from build123d import *

# Parameters (mm, degrees)
F0_W        = 304.8
F0_H        = 304.8
F0_R        = 139.7
F1_DEPTH    = 63.5
F3_D        = 6.35
F2_W        = 38.1
F2_H        = 38.1
F2_R        = 1.5875
F4_DEPTH    = 25.4
F5_T1_DEPTH = 825.5


# Not quite as in the source:
# - a fillet or chamfer that OpenCascade refuses, or shapes differently, is made with other operations: its cross-section is extruded or revolved along the edge and cut away or added


with BuildPart() as f1:
    # F0 (on Top) → F1 (new body)
    with BuildSketch(Plane.XY):
        Rectangle(F0_W, F0_H)
        Circle(F0_R, mode=Mode.SUBTRACT)
    extrude(amount=F1_DEPTH)

    # F3 (through all)
    with Locations(Plane(origin=(0, 152.4, 0), x_dir=(-1, 0, 0), z_dir=(0, 1, 0))):
        with Locations((0, 31.75)):
            Hole(F3_D / 2)

    # F2 (on face) → F4 (cut)
    with BuildSketch(Plane(origin=(0, 152.4, 0), x_dir=(-1, 0, 0), z_dir=(0, 1, 0))):
        with Locations((0, 31.75)):
            Rectangle(F2_W, F2_H)
        with Locations((0, 31.75)):
            Circle(F2_R, mode=Mode.SUBTRACT)
    extrude(amount=-F4_DEPTH, mode=Mode.SUBTRACT)

    # F5: fillet of radius 152.4 on 4 edges, made by hand

    # F5_s2 → F5_t1 (cut)
    with BuildSketch(Plane.XY.offset(-381)):
        with BuildLine():
            ThreePointArc((0, 152.4), (-107.7630734528, 107.7630734528), (-152.4, 0))
            Line((-152.4, 0), (-152.4, 152.4))
            Line((-152.4, 152.4), (0, 152.4))
        make_face()
        with BuildLine():
            ThreePointArc((152.4, 0), (107.7630734528, 107.7630734528), (0, 152.4))
            Line((0, 152.4), (152.4, 152.4))
            Line((152.4, 152.4), (152.4, 0))
        make_face()
        with BuildLine():
            ThreePointArc((152.4, 0), (107.7630734528, -107.7630734528), (0, -152.4))
            Line((0, -152.4), (152.4, -152.4))
            Line((152.4, -152.4), (152.4, 0))
        make_face()
        with BuildLine():
            ThreePointArc((0, -152.4), (-107.7630734528, -107.7630734528), (-152.4, 0))
            Line((-152.4, 0), (-152.4, -152.4))
            Line((-152.4, -152.4), (0, -152.4))
        make_face()
    extrude(amount=F5_T1_DEPTH, mode=Mode.SUBTRACT)


solid = f1.part
Read the model definition and answer for the solid it produces. Units are mm, in the model's axes. A direction names the side the tool comes from. Round coordinates to 2 decimals unless told otherwise and drop trailing zeros. Order: outer loops, then holes, each group sorted by start corner. A loop starts at its lowest first (then second) coordinate and runs counter-clockwise, first axis right, second up. Notation, with made-up numbers: (2.5, -12.5) - (24.5, -12.5) arc R19 cw to (24.5, -7.5) - close; hole circle Ø7 at (65, 38.5). An arc over 180 degrees is marked (long way). Use one line per item in the form item = value. Start each with the question number.
(1) For faces 1 (the face through (67, -123, 0)), 2 (the face through (0, 145, 50.8)), determine the directions among +Z, -Z, +X, -X, +Y, -Y from which every point of the face is accessible in a straight line to the end or side of a thin tool.
(2) Find the intervals of material crossed by line 1 along Z through (x, y) = (0, -145) (3 decimals); line 2 along X through (y, z) = (3, 20); line 3 along X through (y, z) = (-86, 54), in increasing order. Write a range as from..to.
(3) The part is cut by section C-C (z = 58.5). Give the vertices of the cut face in (x, y), then the cut area to 3 significant figures.
(4) Determine the mould class of faces 3 (the face through (67, -123, 63.5)), 4 (the face through (-30.28, -136.38, 31.31)) for opening direction Y: +Y half, -Y half, draft (parallel to the pull), parting line (faces both ways), or undercut.
(5) The part is cut by section A-A (y = 102). Give the vertices of the cut face in (x, z).
(6) The part is cut by section B-B (x = 96). Give the vertices of the cut face in (y, z).
(7) Flat-ended cylindrical pins translate along their axes: pin 1 Ø1 at (y, z) = (120.5, 26.5) entering from +X; pin 2 Ø1.5 at (y, z) = (10.5, 20.5) entering from -X; pin 3 Ø8.5 at (x, z) = (0, 31.75) entering from -Y; pin 4 Ø4 at (y, z) = (6, 6.5) entering from -X. Find the tip coordinate at first contact, or state that the pin passes through.
Checked values:
q1.face_1 = -Z, +X, -X, +Y, -Y
q1.face_2 = +Y
q2.line_1 = 0..28.575, 34.925..63.5
q2.line_2 = -152.37..-139.67, 139.67..152.37
q2.line_3 = -125.82..-110.09, 110.09..125.82
q3.outline = circle Ø304.8 at (0, 0); hole circle Ø279.4 at (0, 0)
q3.area = 11,700 mm^2
q4.face_3 = draft
q4.face_4 = undercut
q5.outline = (-113.23, 0) - (-95.46, 0) - (-95.46, 63.5) - (-113.23, 63.5) - close; (95.46, 0) - (113.23, 0) - (113.23, 63.5) - (95.46, 63.5) - close
q6.outline = (-118.36, 0) - (-101.49, 0) - (-101.49, 63.5) - (-118.36, 63.5) - close; (101.49, 0) - (118.36, 0) - (118.36, 63.5) - (101.49, 63.5) - close
q7.pin_1 = 93.95
q7.pin_2 = -152.09
q7.pin_3 = -152.4
q7.pin_4 = -152.35
